Read the model definition and answer for the solid it produces. Units are mm, in the model's axes. A direction names the side the tool comes from. Coordinates: 2 decimals unless noted, no trailing zeros. Write each loop counter-clockwise with the first axis right and the second up, starting at its lowest first coordinate (ties: lowest second). Pieces come first, ordered by that corner, then holes. Notation, with made-up numbers: M -24,16 L 31,16 A23 cw 31,40 Z; hole C 66.5,-12.75 d4. An arc over 180 degrees is marked long. Write item = value, one per line.
Autodesk Inventor part; units mm, degrees
ref_plane "YZ Plane" through (0, 0, 0) normal (1, 0, 0) x (0, 1, 0)
ref_plane "XZ Plane" through (0, 0, 0) normal (0, 1, 0) x (-1, 0, 0)
ref_plane "XY Plane" through (0, 0, 0) normal (0, 0, 1) x (1, 0, 0)
sketch "Sketch1" plane through (0, 0, 0) normal (0, 0, 1) x (1, 0, 0)
  line L0 (-12.7, -12.7) -> (-12.7, 12.7)
  line L1 (-12.7, 12.7) -> (12.7, 12.7)
  line L2 (12.7, 12.7) -> (12.7, -12.7)
  line L3 (12.7, -12.7) -> (-12.7, -12.7)
  line L4 (-12.7, -12.7) -> (12.7, 12.7) construction
  line L5 (-12.7, 12.7) -> (12.7, -12.7) construction
  line L6 (11.1125, 11.1125) -> (-11.1125, 11.1125)
  line L7 (-11.1125, 11.1125) -> (-11.1125, -11.1125)
  line L8 (-11.1125, -11.1125) -> (11.1125, -11.1125)
  line L9 (11.1125, -11.1125) -> (11.1125, 11.1125)
  point P0 (0, 0)
  dimension "d0" = 25.4
  dimension "d1" = 25.4
  dimension "d2" = 1.5875
extrude "Extrusion1" add sketch "Sketch1" along normal blind 355.6
sketch "Sketch2" plane through (-12.7, 12.7, 0) normal (0, 1, 0) x (1, 0, 0)
  line L0 (25.4, 0) -> (0, 0)
  line L1 (0, 0) -> (0, -355.6)
  line L2 (25.4, -355.6) -> (0, -355.6)
  line L3 (25.4, 0) -> (25.4, -355.6)
  circle A0 centre (12.7, -12.7) radius 2.5781
  circle A1 centre (12.7, -38.1) radius 2.5781
  circle A2 centre (12.7, -63.5) radius 2.5781
  line L4 (1.5875, 0) -> (1.5875, -355.6) construction
  line L5 (1.5875, -177.8) -> (25.4, -177.8) construction
  circle A3 centre (12.7, -342.9) radius 2.5781
  circle A4 centre (12.7, -317.5) radius 2.5781
  circle A5 centre (12.7, -292.1) radius 2.5781
  point P0 (12.7, 0)
  dimension "d5" = 5.1562
  dimension "d6" = 5.1562
  dimension "d7" = 12.7
  dimension "d8" = 25.4
  dimension "d9" = 25.4
  dimension "d10" = 12.7
extrude "Extrusion2" cut sketch "Sketch2" against normal through all contours A0 | A1 | A2 | A3 | A4 | A5
equation "\"d1\" = d0"
properties part number "14in long 1in square tube"
Item 1: Which of the six approach directions +Z, -Z, +X, -X, +Y, -Y give full straight-line access (tool end or side, diameter ignored) to faces 4 (the face through (-11.112, 0, 175)), 5 (the face through (-12.7, 0, 175))?
Worked answers:
face_4 = +Z, -Z
face_5 = +Z, -Z, -X, +Y, -Y
Item 2: A flat-ended cylindrical pin translates along its axis: pin 1 (4.5 mm diameter, centred on x = 0, z = 317.5, fed in from +Y). Find the tip coordinate at first contact, or state that the pin passes through.
Worked answers:
pin_1 = through
Item 3: Find section B-B (y = -5.75). Determine the outline of the cut face in (x, z), and give its area (3 significant figures).
Worked answers:
outline = M -12.7,0 L -11.11,0 L -11.11,355.6 L -12.7,355.6 Z; M 11.11,0 L 12.7,0 L 12.7,355.6 L 11.11,355.6 Z
area = 1,130 mm²
Item 4: Consider line 1 along X through (y, z) = (5.5, 312.5); line 2 along X through (y, z) = (-11.6, 63.5). Determine where each line is inside the solid, lowest interval first. Write a range as from..to.
Worked answers:
line_1 = -12.7..-11.11, 11.11..12.7
line_2 = -12.7..-2.58, 2.58..12.7
Item 5: Find section A-A (z = 305). Determine the outline of the cut face in (x, y).
Worked answers:
outline = M -12.7,-12.7 L 12.7,-12.7 L 12.7,12.7 L -12.7,12.7 Z; hole M -11.11,-11.11 L 11.11,-11.11 L 11.11,11.11 L -11.11,11.11 Z
Item 6: For a pull along X with two mould halves and no side action, classify faces 1 (the face through (0, -12.7, 175)), 2 (the face through (12.7, 0, 175)), 3 (the face through (0, -11.112, 175)) as released by +X, released by -X, zero draft, split by the parting line, or undercut.
Worked answers:
face_1 = zero draft
face_2 = released by +X
face_3 = undercut
